The model under review builds one solid part; all positions refer to its coordinate system, in mm. Face numbers are marked on the shaded views. A direction names the side the tool comes from. Coordinates: 2 decimals unless noted, no trailing zeros. Order: outer loops, then holes, each group sorted by start corner. A loop starts at its lowest first (then second) coordinate and runs counter-clockwise, first axis right, second up.
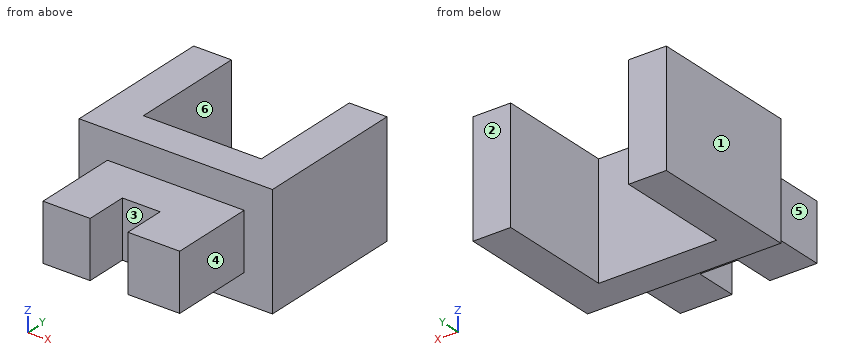
Autodesk Inventor part; units mm, degrees
ref_plane "YZ Plane" through (0, 0, 0) normal (1, 0, 0) x (0, 1, 0)
ref_plane "XZ Plane" through (0, 0, 0) normal (0, 1, 0) x (-1, 0, 0)
ref_plane "XY Plane" through (0, 0, 0) normal (0, 0, 1) x (1, 0, 0)
sketch "Sketch1" plane through (0, 0, 0) normal (0, 0, 1) x (1, 0, 0)
  line L0 (-0.1073, 3.7083) -> (12.3927, 3.7083)
  line L1 (12.3927, 3.7083) -> (12.3927, 0)
  line L2 (12.3927, 0) -> (-0.1073, 0)
  line L3 (-0.1073, 0) -> (-0.1073, 3.7083)
  line L4 (-0.1073, 0) -> (-4.1073, 0)
  line L5 (-4.1073, 0) -> (-4.1073, 16)
  line L6 (-4.1073, 16) -> (-0.1073, 16)
  line L7 (-0.1073, 16) -> (-0.1073, 0)
  line L8 (12.3927, 0) -> (16.3927, 0)
  line L9 (16.3927, 0) -> (16.3927, 16)
  line L10 (16.3927, 16) -> (12.3927, 16)
  line L11 (12.3927, 16) -> (12.3927, 0)
  point P0 (0, 0)
  dimension "d0" = 12.5
  dimension "d1" = 16
  dimension "d2" = 4
  dimension "d3" = 4
extrude "Extrusion1" add sketch "Sketch1" along normal blind 12
sketch "Sketch2" plane through (-4.1073, 0, 0) normal (0, -1, 0) x (1, 0, 0)
  line L0 (0, 12) -> (20.5, 12)
  line L1 (0, 0) -> (20.5, 0)
  line L2 (0, 0) -> (0, 12)
  point P0 (4.1073, 0)
sketch "Sketch3" plane through (-4.1073, 0, 0) normal (0, -1, 0) x (1, 0, 0)
  line L0 (17.5, 3) -> (17.5, 9)
  line L1 (0, 0) -> (20.5, 0)
  line L2 (0, 0) -> (0, 12)
  line L3 (20.5, 0) -> (20.5, 12)
  line L4 (17.5, 3) -> (3, 3)
  line L5 (3, 3) -> (3, 9)
  line L6 (3, 9) -> (17.5, 9)
  line L7 (17.5, 9) -> (17.5, 3)
  point P0 (4.1073, 0)
  dimension "d20" = 3
  dimension "d21" = 3
extrude "Extrusion4" add sketch "Sketch3" along normal blind 4.5
sketch "Sketch5" plane through (-4.1073, -4.5, 0) normal (0, -1, 0) x (1, 0, 0)
  line L0 (3, 3) -> (17.5, 3)
  line L1 (3, 9) -> (17.5, 9)
  line L2 (17.5, 3) -> (12, 3)
  line L3 (12, 3) -> (12, 9)
  line L4 (12, 9) -> (17.5, 9)
  line L5 (17.5, 9) -> (17.5, 3)
  line L6 (3, 3) -> (8, 3)
  line L7 (8, 3) -> (8, 9)
  line L8 (8, 9) -> (3, 9)
  line L9 (3, 9) -> (3, 3)
  point P0 (4.1073, 0)
  dimension "d24" = 4
  dimension "d25" = 5.5
extrude "Extrusion5" add sketch "Sketch5" along normal blind 4.5 contours L9 L1 L7 L0 | L3 L1 L5 L0
properties part number "servo_motor_clip"
(1) For pin 1 Ø2 at (y, z) = (-7.5, 6) entering from +X; pin 2 Ø1.8 at (y, z) = (-5, 6.5) entering from -X; pin 3 Ø1.5 at (x, z) = (8.5, 7) entering from +Y, all flat-tipped, find the tip position at first contact; note any pin that passes through.
A:
pin 1: stops at x = 13.39
pin 2: stops at x = -1.11
pin 3: stops at y = 3.71
(2) We need section C-C, the plane x = 10.25. Write out the cut boundary in (y, z).
A:
outline: (-9, 3) - (0, 3) - (0, 0) - (3.71, 0) - (3.71, 12) - (0, 12) - (0, 9) - (-9, 9) - close
(3) Machinability: for the marked faces 4, 5 and 6, which of the approach directions +Z, -Z, +X, -X, +Y, -Y give a long, thin tool a straight path to every point of the face, cutting with its end or side? Answer none if there is none.
A:
face 4: +Z, -Z, +X, -Y
face 5: +Z, -Z, -X, -Y
face 6: +Z, -Z, +Y
(4) Draft analysis for pull direction X (two halves, no side actions). For the marked faces 1, 2 and 3, state which applies: released by +X, released by -X, zero draft, split by the parting line, or undercut.
A:
face 1: released by -X
face 2: zero draft
face 3: undercut
(5) We need section D-D, the plane z = 10.5. Write out the cut boundary in (x, y), and give its area (3 significant figures).
A:
outline: (-4.11, 0) - (16.39, 0) - (16.39, 16) - (12.39, 16) - (12.39, 3.71) - (-0.11, 3.71) - (-0.11, 16) - (-4.11, 16) - close
area: 174 mm2
(6) We need section B-B, the plane z = 5.5. Write out the cut boundary in (x, y).
A:
outline: (-4.11, 0) - (-1.11, 0) - (-1.11, -9) - (3.89, -9) - (3.89, -4.5) - (7.89, -4.5) - (7.89, -9) - (13.39, -9) - (13.39, 0) - (16.39, 0) - (16.39, 16) - (12.39, 16) - (12.39, 3.71) - (-0.11, 3.71) - (-0.11, 16) - (-4.11, 16) - close
(7) We need section A-A, the plane y = 5.5. Write out the cut boundary in (x, z).
A:
outline: (-4.11, 0) - (-0.11, 0) - (-0.11, 12) - (-4.11, 12) - close; (12.39, 0) - (16.39, 0) - (16.39, 12) - (12.39, 12) - close
(8) Wall thickness on probe 1 along X at (y, z) = (9, 5.5); probe 2 along X at (y, z) = (-5.75, 6); probe 3 along Y at (x, z) = (-1.25, 2): over which ranges is each line inside the solid? List them lowest first.
A:
probe 1: x = -4.11 to -0.11, 12.39 to 16.39
probe 2: x = -1.11 to 3.89, 7.89 to 13.39
probe 3: y = 0 to 16
